Model file for the job. Use its own axes, mm. Round coordinates to 2 decimals unless told otherwise and drop trailing zeros. Loops run counter-clockwise (first coordinate to the right, second up) from the corner with the lowest first, then second, coordinate; pieces in that order, holes last. Notation, with made-up numbers: (-13.5, 47) -> (32.5, 47) arc R22 cw to (32.5, 75) -> close; hole circle Ø11 at (54, -38). An arc over 180 degrees is marked (long way). Use a Markdown table: item, result. Add a question column.
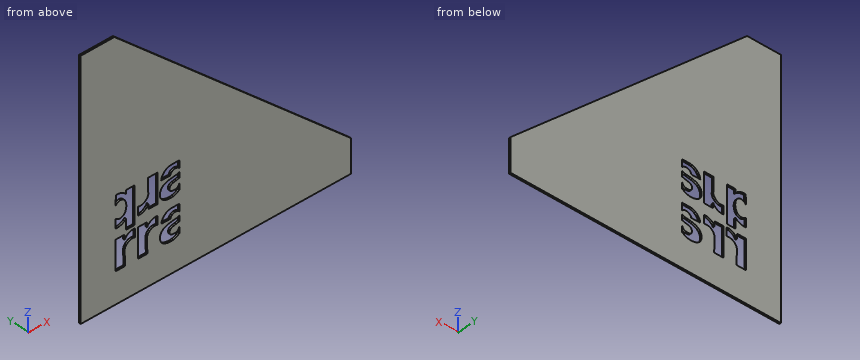
```python
from build123d import *

# Parameters (mm, degrees)
F1_DEPTH = 2


with BuildPart() as f1:
    # F0 (on Front) → F1 (new body)
    with BuildSketch(Plane.XZ):
        Polygon((207.8597095609, 332.3038927495), (207.8597095609, 33.0038927495), (527.8597095609, 33.0038927495), (527.8597095609, 73.0038927495), (247.8597095609, 333.0038927495), (207.8597095609, 333.0038927495), align=None)
        with BuildLine():
            Line((260.350984643, 70.2171021446), (249.2783638935, 70.2171021446))
            Line((249.2783638935, 70.2171021446), (249.2783638935, 105.6249880537))
            Line((249.2783638935, 105.6249880537), (259.907719801, 105.6249880537))
            Line((259.907719801, 105.6249880537), (259.907719801, 99.7129225477))
            ThreePointArc((259.907719801, 99.7129225477), (264.969159541, 104.9981198242), (272.166569839, 106.3205295548))
            Line((272.166569839, 106.3205295548), (272.166569839, 96.3221633181))
            ThreePointArc((272.166569839, 96.3221633181), (264.4266251898, 95.3581367621), (259.9412812379, 88.9770882584))
            Line((259.9412812379, 88.9770882584), (260.350984643, 70.2171021446))
        make_face(mode=Mode.SUBTRACT)
        with BuildLine():
            ThreePointArc((286.3925668235, 99.7295484954), (291.4540065635, 105.0147457719), (298.6514168615, 106.3371555025))
            Line((298.6514168615, 106.3371555025), (298.6514168615, 96.3387892658))
            ThreePointArc((298.6514168615, 96.3387892658), (290.9114722123, 95.3747627098), (286.4261282604, 88.9937142061))
            Line((286.4261282604, 88.9937142061), (286.8358316655, 70.2337280923))
            Line((286.8358316655, 70.2337280923), (275.763210916, 70.2337280923))
            Line((275.763210916, 70.2337280923), (275.763210916, 105.6416140014))
            Line((275.763210916, 105.6416140014), (286.3925668235, 105.6416140014))
            Line((286.3925668235, 105.6416140014), (286.3925668235, 99.7295484954))
        make_face(mode=Mode.SUBTRACT)
        with BuildLine():
            Line((324.8531874271, 80.6576142285), (324.8531874271, 72.9894021723))
            add(Edge.make_bspline(
                [(324.8531874271, 93.2830700848), (323.3065188743, 92.0353198263), (319.5932504041, 91.5074140824), (305.76812214, 90.3356227603), (300.2660508817, 80.3600298922), (304.3588181672, 69.9638702682), (318.5536418728, 68.5542730887), (322.0696986329, 71.5322612124), (324.8531874271, 72.9894021723)],
                knots=[0, 0, 0, 0, 0.1282549597, 0.3235779421, 0.4933166916, 0.6588260023, 0.8480719548, 1, 1, 1, 1], degree=3))
            Line((324.8531874271, 93.2830700848), (324.8531874271, 86.6217890952))
            add(Edge.make_bspline(
                [(324.8531874271, 80.6576142285), (324.3853881763, 79.3716732666), (323.4463072091, 76.6838402752), (318.0274043762, 75.8320101397), (313.0517233961, 76.8842047893), (312.8862075691, 83.1667071186), (318.065998571, 85.3140545113), (321.9671157982, 85.6164060676), (324.8531874271, 86.6217890952)],
                knots=[0, 0, 0, 0, 0.1467139352, 0.3148344078, 0.4723324727, 0.6349882053, 0.7976765175, 1, 1, 1, 1], degree=3))
        make_face(mode=Mode.SUBTRACT)
        with BuildLine():
            Line((316.0905669231, 106.2228459891), (324.8531874271, 106.1858685351))
            Line((324.8531874271, 106.1858685351), (324.8531874271, 97.3470781765))
            ThreePointArc((324.8531874271, 97.3470781765), (318.6136208517, 99.4559091904), (313.9553243844, 94.7997698758))
            Line((313.9553243844, 94.7997698758), (303.3299023836, 94.9093083117))
            ThreePointArc((303.3299023836, 94.9093083117), (307.550022404, 103.002604489), (316.0905669231, 106.2228459891))
        make_face(mode=Mode.SUBTRACT)
        with BuildLine():
            Line((271.8778838503, 154.6828896542), (271.8778838503, 110.1980508108))
            Line((271.8778838503, 110.1980508108), (261.5694468009, 110.1980508108))
            Line((261.5694468009, 110.1980508108), (261.5694468009, 122.6266548772))
            ThreePointArc((261.5694468009, 122.6266548772), (256.0058228238, 118.7745070428), (249.2798035133, 118.0304513116))
            Line((249.2798035133, 118.0304513116), (249.2798035133, 129.026845171))
            ThreePointArc((249.2798035133, 129.026845171), (255.1291713772, 126.67333299), (260.419606148, 130.1034093638))
            ThreePointArc((260.419606148, 130.1034093638), (261.9283811203, 136.8586272736), (260.419606148, 143.6138451834))
            ThreePointArc((260.419606148, 143.6138451834), (254.8736584473, 146.8446188485), (249.3277107465, 143.6138451834))
            Line((249.3277107465, 143.6138451834), (249.5063905704, 155.1215500374))
            ThreePointArc((249.5063905704, 155.1215500374), (256.2156097253, 154.2198410632), (261.5694468009, 150.0770003338))
            Line((261.5694468009, 150.0770003338), (261.5694468009, 154.6828896542))
            Line((261.5694468009, 154.6828896542), (271.8778838503, 154.6828896542))
        make_face(mode=Mode.SUBTRACT)
        with BuildLine():
            Line((298.6336936343, 119.2762107392), (288.0043377268, 119.2762107392))
            Line((288.0043377268, 119.2762107392), (288.0043377268, 125.1882762452))
            ThreePointArc((288.0043377268, 125.1882762452), (282.9428979868, 119.9030789686), (275.7454876888, 118.5806692381))
            Line((275.7454876888, 118.5806692381), (275.7454876888, 128.5790354748))
            ThreePointArc((275.7454876888, 128.5790354748), (283.485432338, 129.5430620307), (287.9707762899, 135.9241105345))
            Line((287.9707762899, 135.9241105345), (287.5610728848, 154.6840966483))
            Line((287.5610728848, 154.6840966483), (298.6336936343, 154.6840966483))
            Line((298.6336936343, 154.6840966483), (298.6336936343, 119.2762107392))
        make_face(mode=Mode.SUBTRACT)
        with BuildLine():
            add(Edge.make_bspline(
                [(324.7558644524, 141.9059485932), (323.2091958996, 140.6581983347), (319.4959274294, 140.1302925908), (305.6707991653, 138.9585012686), (300.168727907, 128.9829084005), (304.2614951926, 118.5867487766), (318.4563188981, 117.1771515971), (321.9723756583, 120.1551397208), (324.7558644524, 121.6122806807)],
                knots=[0, 0, 0, 0, 0.1282549597, 0.3235779421, 0.4933166916, 0.6588260023, 0.8480719548, 1, 1, 1, 1], degree=3))
            Line((324.7558644524, 141.9059485932), (324.7558644524, 135.2446676035))
            add(Edge.make_bspline(
                [(324.7558644524, 129.2804927369), (324.2880652016, 127.9945517749), (323.3489842345, 125.3067187836), (317.9300814016, 124.4548886481), (312.9544004215, 125.5070832977), (312.7888845944, 131.7895856269), (317.9686755963, 133.9369330196), (321.8697928236, 134.239284576), (324.7558644524, 135.2446676035)],
                knots=[0, 0, 0, 0, 0.1467139352, 0.3148344078, 0.4723324727, 0.6349882053, 0.7976765175, 1, 1, 1, 1], degree=3))
            Line((324.7558644524, 129.2804927369), (324.7558644524, 121.6122806807))
        make_face(mode=Mode.SUBTRACT)
        with BuildLine():
            Line((324.7558644524, 154.8087470435), (324.7558644524, 145.9699566849))
            ThreePointArc((324.7558644524, 145.9699566849), (318.516297877, 148.0787876987), (313.8580014098, 143.4226483841))
            Line((313.8580014098, 143.4226483841), (303.2325794089, 143.5321868201))
            ThreePointArc((303.2325794089, 143.5321868201), (307.4526994293, 151.6254829974), (315.9932439484, 154.8457244975))
            Line((315.9932439484, 154.8457244975), (324.7558644524, 154.8087470435))
        make_face(mode=Mode.SUBTRACT)
    extrude(amount=F1_DEPTH)


solid = f1.part
```
1) Pin check, flat tips, straight feed: pin 1 Ø1 at (y, z) = (-1.5, 116.5) entering from +X; pin 2 Ø4 at (x, z) = (448, 144.5) entering from +Y; pin 3 Ø1 at (y, z) = (-1, 121.5) entering from +X; pin 4 Ø1 at (x, y) = (294.5, -1) entering from +Z. Stop position of each tip, or through.
2) Cut at C-C on x = 444. Write the cut outline in (y, z), and give its area (3 significant figures).
3) Cut at A-A on y = -1.05. Count the separate pieces of the cut face and the enclosed holes in it, and give its area (3 significant figures).
4) Cut at B-B on z = 202. Write the cut outline in (x, y).
5) Wall check: probe 1 along Z at (x, y) = (279, -0.25); probe 2 along Z at (x, y) = (264, -1.9); probe 3 along Z at (x, y) = (307, -1). Give the ranges that are in metal, low to high. Write a range as from..to.
Established:
| question | item | result |
|---|---|---|
| 1 | pin 1 | stops at x = 481.56 |
| 1 | pin 2 | stops at y = 0 |
| 1 | pin 3 | stops at x = 476.17 |
| 1 | pin 4 | stops at z = 290.16 |
| 2 | outline | (-2, 33) -> (0, 33) -> (0, 150.87) -> (-2, 150.87) -> close |
| 2 | area | 236 mm^2 |
| 3 | separate pieces | 1 |
| 3 | enclosed holes | 8 |
| 3 | area | 56,400 mm^2 |
| 4 | outline | (207.86, -2) -> (388.94, -2) -> (388.94, 0) -> (207.86, 0) -> close |
| 5 | probe 1 | z = 33..70.23, 105.64..118.6, 128.18..304.09 |
| 5 | probe 2 | z = 33..95.09, 104.41..110.2, 154.68..318.02 |
| 5 | probe 3 | z = 33..71.01, 88.62..94.87, 102.49..119.58, 137.3..143.49, 151.2..278.09 |
